Part model, mm, in its own coordinate system. Face numbers are marked on the shaded views. Round coordinates to 2 decimals unless told otherwise and drop trailing zeros. Order: outer loops, then holes, each group sorted by start corner. A loop starts at its lowest first (then second) coordinate and runs counter-clockwise, first axis right, second up. Notation, with made-up numbers: M 44.25,53.5 L 103.25,53.5 A29 cw 103.25,87.5 Z; hole C 72,36.5 d11. An arc over 180 degrees is marked long. Write each question's results on one line, items separated by ' | '. Start each with the question number.
1. Band-saw the part on D-D, the plane z = -60.5. List the corners of the cut face in (x, y).
2. Two-plate mould, pull along Z, no slides. Class the marked faces 1 and 2: +Z half, -Z half, draft (parallel to the pull), parting line (faces both ways), or undercut.
3. Drop flat-ended pins along their axis: pin 1 Ø0.6 at (y, z) = (-70, -71.5) entering from +X; pin 2 Ø2 at (x, y) = (-55, -79) entering from -Z. Give the stop position or say it passes through.
4. Band-saw the part on B-B, the plane y = -77. List the corners of the cut face in (x, z).
5. Probe L1, parallel to X at y = -75, z = -68.25; L2, parallel to Z at x = -55.2, y = -82.5; L3, parallel to Z at x = -55.3, y = -83.5. List the from-to ranges inside material, lowest first. Write a range as [from, to].
6. Band-saw the part on C-C, the plane z = -67.25. List the corners of the cut face in (x, y), then the cut area to 3 significant figures.
7. Band-saw the part on A-A, the plane x = -55.75. List the corners of the cut face in (y, z).
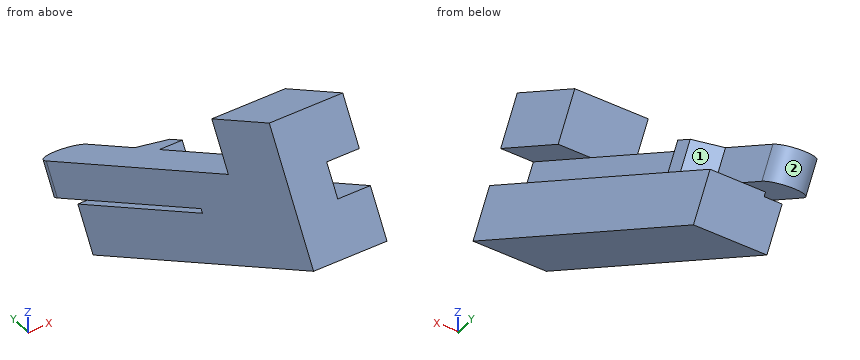
```python
from build123d import *

# Parameters (mm, degrees)
PAD022_DEPTH            = 2
BOX028_W                = 10
BOX028_H                = 4.5
BOX028_DEPTH            = 3
PAD023_DEPTH            = 13
PAD024_DEPTH            = 1.8
BOX029_W                = 6
BOX029_H                = 4.5
BOX029_DEPTH            = 3
BODY012_ROLL_ANGLE      = -0.000328
BODY012_PITCH_ANGLE     = 30.004371
BODY012_PLACEMENT_ANGLE = 89.998778


with BuildPart() as body012:
    # Sketch042 → Pad022 (new body)
    with BuildSketch(Plane(origin=(0, -0.1, 0.2), x_dir=(1, 0, 0), z_dir=(0, 0, 1))):
        with BuildLine():
            Line((24, -2.5), (-1, -2.5))
            Line((-1, -2.5), (-1, 0))
            Line((24, 0), (-1, 0))
            ThreePointArc((24, -2.5), (25.25, -1.25), (24, 0))
        make_face()
    extrude(amount=-PAD022_DEPTH)

    # Box028 → Box028 (join)
    with BuildSketch(Plane(origin=(-1, 1.9, -1.8), x_dir=(1, 0, 0), z_dir=(0, 0, -1))):
        with Locations((5, 2.25)):
            Rectangle(BOX028_W, BOX028_H)
    extrude(amount=BOX028_DEPTH)

    # Sketch043 (on Plane of DatumPlane011) → Pad023 (join)
    with BuildSketch(Plane(origin=(9, -2.6, -4.8), x_dir=(0, 0, 1), z_dir=(1, 0, 0))):
        Polygon((0, 0), (0, -4.5), (3, -4.5), (3, -1.1), (2.75, -1.1), (2.75, 0), align=None)
    extrude(amount=PAD023_DEPTH)

    # Sketch044 (on Plane of DatumPlane002) → Pad024 (join)
    with BuildSketch(Plane.XY.offset(0.2)):
        Polygon((16.45, -0.1), (16.45, 1.3), (17.75, 1.3), (19.05, -0.1), align=None)
    extrude(amount=-PAD024_DEPTH)

    # Box029 → Box029 (join)
    with BuildSketch(Plane(origin=(-1, -2.6, 0.2), x_dir=(1, 0, 0), z_dir=(0, 0, 1))):
        with Locations((3, 2.25)):
            Rectangle(BOX029_W, BOX029_H)
    extrude(amount=BOX029_DEPTH)


with BuildPart() as body012_1:
    # Body012 roll: moved
    add(body012.part.rotate(Axis((0, 0, 0), (1, 0, 0)), BODY012_ROLL_ANGLE))


with BuildPart() as body012_2:
    # Body012 pitch: moved
    add(body012_1.part.rotate(Axis((0, 0, 0), (0, 1, 0)), BODY012_PITCH_ANGLE))


with BuildPart() as body012_3:
    # Body012 placement: moved
    add(body012_2.part.moved(Location((-34.500058, -84.760808, -62.025399))).rotate(Axis((-34.500058, -84.760808, -62.025399), (0, 0, 1)), BODY012_PLACEMENT_ANGLE))


with BuildPart() as body_mirrored:
    # mirror: instance of Body012
    add(body012_3.part.mirror(Plane(origin=(-11, 23.3, 0), x_dir=(0, 1, 0), z_dir=(-1, 0, 0))))


with BuildPart() as body_mirrored_1:
    # mirror placement: moved
    add(body_mirrored.part.moved(Location((-69, 0, 0))))


solid = body_mirrored_1.part
```
Solution:
1) outline: M -59.1,-85.03 L -54.6,-85.03 L -54.6,-81 L -59.1,-81 Z
2) face 1: undercut | face 2: -Z half
3) pin 1: x = -55.2 | pin 2: z = -71.47
4) outline: M -59.1,-72.05 L -54.6,-72.05 L -54.6,-68.59 L -56.6,-68.59 L -56.6,-66.28 L -59.1,-66.28 L -59.1,-68.59 L -58,-68.59 L -58,-68.87 L -59.1,-68.87 Z
5) L1: [-59.1, -56.6] | L2: [-68.87, -65.41], [-63.1, -59.64] | L3: [-68.3, -64.83], [-62.52, -59.06]
6) outline: M -59.1,-85.31 L -54.6,-85.31 L -54.6,-79.31 L -56.6,-79.31 L -56.6,-75.31 L -59.1,-75.31 Z | area: 37.0 mm^2
7) outline: M -88.03,-65.68 L -68.11,-77.18 L -66.61,-74.59 L -86.53,-63.08 Z; M -85.53,-61.35 L -80.33,-64.35 L -78.83,-61.75 L -84.03,-58.75 Z; M -71.32,-71.64 L -69.75,-72.54 L -68.85,-70.98 L -70.42,-70.08 Z
